The model under review builds one solid part; all positions refer to its coordinate system, in mm. Give positions to 0.01 mm unless a question says otherwise; leave off trailing zeros. Loops run counter-clockwise (first coordinate to the right, second up) from the corner with the lowest first, then second, coordinate; pieces in that order, holes last. Notation, with made-up numbers: M -34,71.5 L 25,71.5 A26 cw 25,110.5 Z; hole C 85,-21 d7. An arc over 180 degrees is marked long. One line per item, written item: value. Start each with the question number.
Q1. We need section B-B on x = -111.5. Write out the cut boundary in (y, z), plus the area to 4 significant figures.
Q2. For pin 1 (1.8 mm diameter, centred on x = -214, z = -46, fed in from +Y); pin 2 (0.9 mm diameter, centred on x = 32.5, z = 11.5, fed in from -Y); pin 3 (5.5 mm diameter, centred on y = -3.5, z = 23, fed in from -X); pin 4 (2.5 mm diameter, centred on x = 88, z = -19.5, fed in from +Y), all flat-tipped, find the tip position at first contact; note any pin that passes through.
Q3. To check wall thickness, follow line 1 along X through (y, z) = (-3.7, -16); line 2 along Z through (x, y) = (-52.5, -5.25); line 3 along X through (y, z) = (-6.55, -62). State the ranges of each line that lie inside material, in increasing order. Write a range as from..to.
Q4. We need section C-C on z = 32. Write out the cut boundary in (x, y).
Q5. We need section A-A on x = 4. Write out the cut boundary in (y, z), plus the area to 3 significant figures.
```python
from build123d import *

# Parameters (mm, degrees)
SKETCH1_W           = 400
SKETCH1_H           = 360
BOSS_EXTRUDE1_DEPTH = 10
CUT_EXTRUDE1_DEPTH  = 285.429253067
CUT_EXTRUDE2_DEPTH  = 2
SKETCH5_R           = 1.5
CUT_EXTRUDE3_DEPTH  = 3
CUT_EXTRUDE6_DEPTH  = 5
CUT_EXTRUDE7_DEPTH  = 5
SKETCH11_R          = 1.5
CUT_EXTRUDE8_DEPTH  = 285.297379517
SKETCH14_W          = 160
SKETCH14_H          = 10
CUT_EXTRUDE9_DEPTH  = 5
SKETCH15_W          = 5
SKETCH15_H          = 295.150358454
SKETCH15_W_2        = 280
SKETCH15_H_2        = 5
CUT_EXTRUDE10_DEPTH = 5
CHAMFER2_SIZE       = 1


with BuildPart() as part:
    # Sketch1 → Boss-Extrude1 (new body)
    with BuildSketch(Plane(origin=(0, 0, 0), x_dir=(1, 0, 0), z_dir=(0, 1, 0))):
        with Locations((-20, 0)):
            Rectangle(SKETCH1_W, SKETCH1_H)
    extrude(amount=-BOSS_EXTRUDE1_DEPTH)

    # Sketch3 → Cut-Extrude1 (cut, through all)
    with BuildSketch(Plane(origin=(0, 0, 0), x_dir=(1, 0, 0), z_dir=(0, 1, 0))):
        with BuildLine():
            Line((-45, 60), (25, 60))
            ThreePointArc((25, 60), (28.535533906, 58.535533906), (30, 55))
            Line((30, 55), (30, -5))
            ThreePointArc((30, -5), (28.535533906, -8.535533906), (25, -10))
            Line((25, -10), (-45, -10))
            ThreePointArc((-45, -10), (-48.535533906, -8.535533906), (-50, -5))
            Line((-50, -5), (-50, 55))
            ThreePointArc((-50, 55), (-48.535533906, 58.535533906), (-45, 60))
        make_face()
    extrude(amount=-CUT_EXTRUDE1_DEPTH, mode=Mode.SUBTRACT)

    # Sketch4 → Cut-Extrude2 (cut)
    with BuildSketch(Plane.XZ.offset(10)):
        with BuildLine():
            Line((-52, 18), (32, 18))
            ThreePointArc((32, 18), (36.242640687, 16.242640687), (38, 12))
            Line((38, 12), (38, -62))
            ThreePointArc((38, -62), (36.242640687, -66.242640687), (32, -68))
            Line((32, -68), (-52, -68))
            ThreePointArc((-52, -68), (-56.242640687, -66.242640687), (-58, -62))
            Line((-58, -62), (-58, 12))
            ThreePointArc((-58, 12), (-56.242640687, 16.242640687), (-52, 18))
        make_face()
    extrude(amount=-CUT_EXTRUDE2_DEPTH, mode=Mode.SUBTRACT)

    # Sketch5 → Cut-Extrude3 (cut)
    with BuildSketch(Plane.XZ.offset(8)):
        with Locations(Location((32, 12, 0), (0, 0, 270))):
            Circle(SKETCH5_R)
        with Locations(Location((-52, 12, 0), (0, 0, 270))):
            Circle(SKETCH5_R)
        with Locations(Location((32, -62, 0), (0, 0, 270))):
            Circle(SKETCH5_R)
        with Locations(Location((-52, -62, 0), (0, 0, 270))):
            Circle(SKETCH5_R)
    extrude(amount=-CUT_EXTRUDE3_DEPTH, mode=Mode.SUBTRACT)

    # Sketch9 → Cut-Extrude6 (cut)
    with BuildSketch(Plane(origin=(0, -10, 0), x_dir=(1, 0, 0), z_dir=(0, 1, 0))):
        with BuildLine():
            Line((-220, 50), (-195, 50))
            ThreePointArc((-195, 50), (-191.464466094, 48.535533906), (-190, 45))
            Line((-190, 45), (-190, -45))
            ThreePointArc((-190, -45), (-191.464466094, -48.535533906), (-195, -50))
            Line((-195, -50), (-220, -50))
            Line((-220, -50), (-220, 50))
        make_face()
    extrude(amount=CUT_EXTRUDE6_DEPTH, mode=Mode.SUBTRACT)

    # Sketch10 → Cut-Extrude7 (cut)
    with BuildSketch(Plane(origin=(0, -5, 0), x_dir=(-1, 0, 0), z_dir=(0, -1, 0))):
        with BuildLine():
            Line((220, 42), (220, -42))
            Line((220, -42), (203, -42))
            ThreePointArc((203, -42), (199.464466094, -40.535533906), (198, -37))
            Line((198, -37), (198, 37))
            ThreePointArc((198, 37), (199.464466094, 40.535533906), (203, 42))
            Line((203, 42), (220, 42))
        make_face()
    extrude(amount=-CUT_EXTRUDE7_DEPTH, mode=Mode.SUBTRACT)

    # Sketch11 → Cut-Extrude8 (cut, through all)
    with BuildSketch(Plane(origin=(0, -5, 0), x_dir=(-1, 0, 0), z_dir=(0, -1, 0))):
        with Locations(Location((214, 46, 0), (0, 0, 90))):
            Circle(SKETCH11_R)
        with Locations(Location((194, 16, 0), (0, 0, 90))):
            Circle(SKETCH11_R)
        with Locations(Location((196.5, 44.75, 0), (0, 0, 90))):
            Circle(SKETCH11_R)
        with Locations(Location((196.5, -44.75, 0), (0, 0, 270))):
            Circle(SKETCH11_R)
        with Locations(Location((194, -16, 0), (0, 0, 270))):
            Circle(SKETCH11_R)
        with Locations(Location((214, -46, 0), (0, 0, 270))):
            Circle(SKETCH11_R)
    extrude(amount=-CUT_EXTRUDE8_DEPTH, mode=Mode.SUBTRACT)

    # Sketch14 → Cut-Extrude9 (cut)
    with BuildSketch(Plane(origin=(0, 0, 0), x_dir=(1, 0, 0), z_dir=(0, 1, 0))):
        with Locations((-118, 0)):
            Rectangle(SKETCH14_W, SKETCH14_H)
    extrude(amount=-CUT_EXTRUDE9_DEPTH, mode=Mode.SUBTRACT)

    # Sketch15 → Cut-Extrude10 (cut)
    with BuildSketch(Plane(origin=(0, 0, 0), x_dir=(1, 0, 0), z_dir=(0, 1, 0))):
        with Locations((-20, 7.575179227)):
            Rectangle(SKETCH15_W, SKETCH15_H)
        with Locations((0, 20)):
            Rectangle(SKETCH15_W_2, SKETCH15_H_2)
    extrude(amount=-CUT_EXTRUDE10_DEPTH, mode=Mode.SUBTRACT)

    # Chamfer2
    chamfer2_edges = [part.edges().sort_by_distance(p)[0] for p in [
        (-214, 0, 44.5),
        (-194, 0, 14.5),
        (-196.5, 0, 43.25),
        (-196.5, 0, -43.25),
        (-194, 0, -14.5),
        (-214, 0, -44.5),
    ]]
    chamfer(chamfer2_edges, length=CHAMFER2_SIZE)


solid = part.part
```
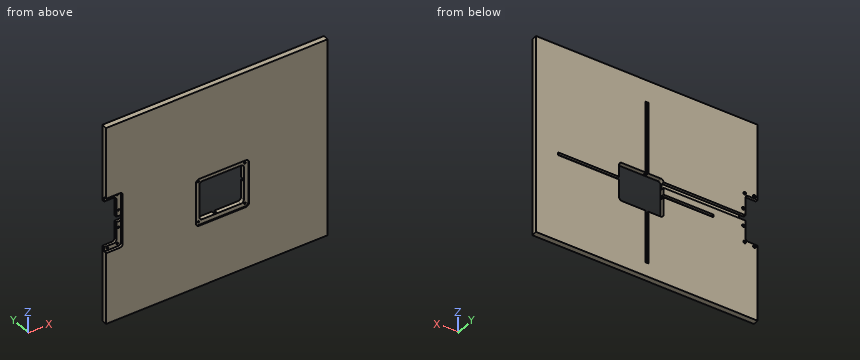
Solved:
1. outline: M -10,-180 L 0,-180 L 0,-22.5 L -5,-22.5 L -5,-17.5 L 0,-17.5 L 0,-5 L -5,-5 L -5,5 L 0,5 L 0,180 L -10,180 Z
1. area: 3,525 mm2
2. pin 1: through
2. pin 2: y = -5
2. pin 3: x = -198
2. pin 4: y = -5
3. line 1: -198..-195.5, -192.5..-50, 30..180
3. line 2: -180..-63.41, -60.59..10.59, 13.41..180
3. line 3: -220..-53.5, -50.5..30.5, 33.5..180
4. outline: M -198,-5 L -190,-5 L -190,-10 L 180,-10 L 180,0 L -17.5,0 L -17.5,-5 L -22.5,-5 L -22.5,0 L -198,0 Z
5. outline: M -10,-180 L 0,-180 L 0,-60 L -8,-60 L -8,-68 L -10,-68 Z; M -10,18 L -8,18 L -8,10 L 0,10 L 0,180 L -10,180 Z
5. area: 2,870 mm2
